Answer from the drawing. Dimensions are ordinates in mm from the lowest x, y and z of the part. A direction names the side the tool comes from. Round coordinates to 2 decimals unless told otherwise and drop trailing zeros. Write each loop counter-clockwise with the first axis right and the second up, starting at its lowest first coordinate (ties: lowest second). Pieces come first, ordered by that corner, then holes.
1. Determine the mould class of the marked faces 1, 2 and 3 for opening direction Z: pulls with the +Z half, pulls with the -Z half, needs draft (parallel to the pull), parting line crosses it, or undercut.
2. Find section B-B (z = 12). Write down the section's boundary in (x, y).
3. Find section A-A (y = 20). Write down the section's boundary in (x, z), and give its area (3 significant figures).
4. Flat-ended cylindrical pins translate along their axes: pin 1 Ø8 at (x, z) = (10, 23.5) entering from +Y; pin 2 Ø11 at (x, y) = (11.5, 20.5) entering from +Z; pin 3 Ø1.5 at (x, y) = (15.5, 27.5) entering from -Z; pin 4 Ø11 at (y, z) = (18.5, 3.5) entering from +X. Find the tip coordinate at first contact, or state that the pin passes through.
5. Find section D-D (x = 2.5). Write down the section's boundary in (y, z), and give its area (3 significant figures).
6. Straight lines are drawn through the part: probe 1 along X at (y, z) = (17.5, 57); probe 2 along Z at (x, y) = (6.25, 14); probe 3 along Y at (x, z) = (4.25, 66). For each, find the intervals that lie inside material, in ascending order.
7. A tool of negligible diameter and unlimited length cuts with its end or side. For the marked faces 4, 5, 6 and 7, from which of +Z, -Z, +X, -X, +Y, -Y can it reach the whole face along a straight path? Write none if from no direction.
8. Find section C-C (y = 36). Write down the section's boundary in (x, z), and give its area (3 significant figures).
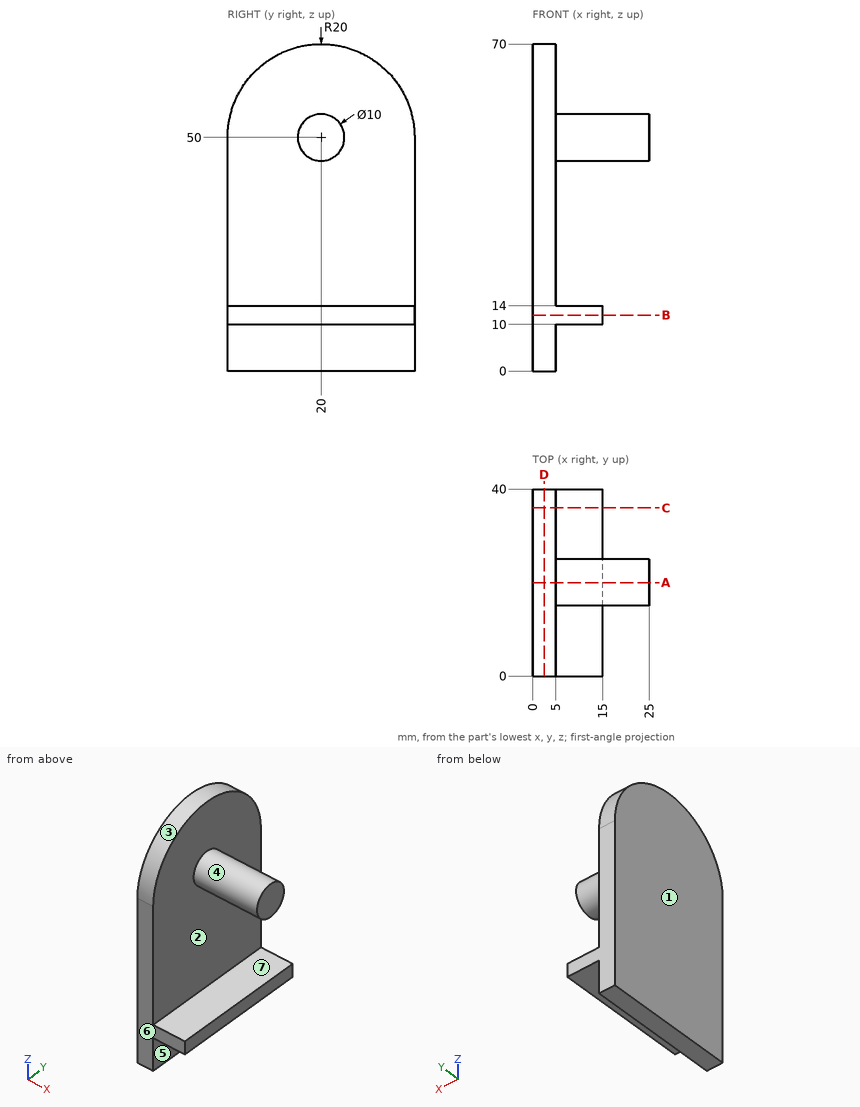
Worked answers:
1. face 1: needs draft
1. face 2: undercut
1. face 3: pulls with the +Z half
2. outline: (0, 0) - (15, 0) - (15, 40) - (0, 40) - close
3. outline: (0, 0) - (5, 0) - (5, 10) - (15, 10) - (15, 14) - (5, 14) - (5, 45) - (25, 45) - (25, 55) - (5, 55) - (5, 70) - (0, 70) - close
3. area: 590 mm2
4. pin 1: passes through
4. pin 2: stops at z = 55
4. pin 3: stops at z = 10
4. pin 4: stops at x = 5
5. outline: (0, 0) - (40, 0) - (40, 50) arc R20 ccw to (0, 50) - close
5. area: 2,630 mm2
6. probe 1: x = 0 to 5
6. probe 2: z = 10 to 14
6. probe 3: y = 8 to 32
7. face 4: +X
7. face 5: -Z, +X, +Y, -Y
7. face 6: +Z, -Z, +X, -X, -Y
7. face 7: +X, +Y, -Y
8. outline: (0, 0) - (5, 0) - (5, 10) - (15, 10) - (15, 14) - (5, 14) - (5, 62) - (0, 62) - close
8. area: 350 mm2
